from build123d import *

# Parameters (mm, degrees)
F0_R     = 1.85
F1_DEPTH = 2.5


# Not quite as in the source:
# - a feature names something its author has since deleted; it is built from what else it names


with BuildPart() as f1:
    # F0 (on Front) → F1 (new body, symmetric)
    with BuildSketch(Plane.XZ):
        with BuildLine():
            Line((4.1206300291, 6.8571428571), (-55.8793699709, 42.9126556118))
            ThreePointArc((-55.8793699709, 42.9126556118), (-63.9392232589, 43.0184517976), (-68, 36.0555127546))
            Line((-68, 36.0555127546), (-68, -23.9444872454))
            Line((-68, -23.9444872454), (8, -23.9444872454))
            Line((8, -23.9444872454), (8, 0))
            ThreePointArc((8, 0), (6.962939043, 3.9392232589), (4.1206300291, 6.8571428571))
        make_face()
        Circle(F0_R, mode=Mode.SUBTRACT)
        with Locations((-60, 36.0555127546)):
            Circle(F0_R, mode=Mode.SUBTRACT)
    extrude(amount=F1_DEPTH, both=True)


solid = f1.part
Work out the finished part from the listing and answer in its coordinate system (mm). Round coordinates to 2 decimals unless told otherwise and drop trailing zeros. Order: outer loops, then holes, each group sorted by start corner. A loop starts at its lowest first (then second) coordinate and runs counter-clockwise, first axis right, second up. Notation, with made-up numbers: M 52,87 L 75,87 A18 cw 75,114 Z; hole C -28.5,49.5 d4. An arc over 180 degrees is marked long. Put each result on its own line as item: value. Start each with the question number.
Q1. Section A-A, the plane x = -60 is taken. Write down the section's boundary in (y, z), and give its area (4 significant figures).
Q2. Straight lines are drawn through the part: L1, parallel to Z at x = -60, y = -0.25; L2, parallel to Z at x = 0, y = 1.25; L3, parallel to X at y = 0.35, z = -1. For each, find the intervals that lie inside material, in ascending order. Write a range as [from, to].
Q3. For a pull along X with two mould halves and no side action, classify faces 1 (the cylindrical face through (-61.36, 0.04, 37.31)), 2 (the cylindrical face through (-0.401, 0.035, -1.806)), 3 (the flat face through (-68, 0, 6)), 4 (the flat face through (-25.459, -0.035, 24.633)) as pulls with the +X half, pulls with the -X half, needs draft (parallel to the pull), parting line crosses it, or undercut.
Q4. A flat-ended cylindrical pin translates along its axis: pin 1 (3 mm diameter, centred on x = -45.5, y = -2, fed in from +Z). Find the tip coordinate at first contact, or state that the pin passes through.
Q5. Section C-C, the plane x = 0 is taken. Write down the section's boundary in (y, z).
Q6. Section D-D, the plane z = 39.5 is taken. Write down the section's boundary in (x, y).
Q7. Section B-B, the plane y = 1.2 is taken. Write down the section's boundary in (x, z).
Findings below:
1. outline: M -2.5,-23.94 L 2.5,-23.94 L 2.5,34.21 L -2.5,34.21 Z; M -2.5,37.91 L 2.5,37.91 L 2.5,44.06 L -2.5,44.06 Z
1. area: 321.5 mm^2
2. L1: z = [-23.94, 34.21], [37.91, 44.06]
2. L2: z = [-23.94, -1.85], [1.85, 9.33]
2. L3: x = [-68, -1.56], [1.56, 8]
3. face 1: undercut
3. face 2: undercut
3. face 3: pulls with the -X half
3. face 4: pulls with the +X half
4. pin 1: stops at z = 37.58
5. outline: M -2.5,-23.94 L 2.5,-23.94 L 2.5,-1.85 L -2.5,-1.85 Z; M -2.5,1.85 L 2.5,1.85 L 2.5,9.33 L -2.5,9.33 Z
6. outline: M -67.22,-2.5 L -50.2,-2.5 L -50.2,2.5 L -67.22,2.5 Z
7. outline: M -68,-23.94 L 8,-23.94 L 8,0 A8 ccw 4.12,6.86 L -55.88,42.91 A8 ccw -68,36.06 Z; hole C -60,36.06 d3.7; hole C 0,0 d3.7
